Print and shaded views of the part. All mm, measured from the part's lowest x, y and z. A direction names the side the tool comes from. Round coordinates to 2 decimals unless told otherwise and drop trailing zeros. Write each loop counter-clockwise with the first axis right and the second up, starting at its lowest first coordinate (ties: lowest second). Pieces come first, ordered by that corner, then holes. Notation, with made-up numbers: M -4,7.5 L 11,7.5 A20 cw 11,41.5 Z; hole C 30.5,26 d8. An arc over 180 degrees is marked long. Write item = value, one per line. Start each with the question number.
Q1. Tool access for the marked faces 1 and 2: list every direction of +Z, -Z, +X, -X, +Y, -Y with a clear straight run to the whole face (end or side of a thin tool).
Q2. Drop flat-ended pins along their axis: P1, Ø2, axis at x = 270, y = 35.5, coming from the -Z side; P2, Ø12, axis at x = 170, y = 78.5, coming from the -Z side; P3, Ø13.5, axis at x = 363.5, y = 60.5, coming from the +Z side; P4, Ø10, axis at x = 107, z = 97.5, coming from the +Y side. Give the stop position or say it passes through.
Q3. Band-saw the part on D-D on z = 34.5. Write the cut outline in (x, y), plus the area to 3 significant figures.
Q4. Band-saw the part on C-C on x = 385. Write the cut outline in (y, z), plus the area to 3 significant figures.
Q5. Band-saw the part on A-A on z = 60. Write the cut outline in (x, y), plus the area to 3 significant figures.
Q6. Probe L1, parallel to X at y = 36, z = 5.5; L2, parallel to X at y = 49, z = 74; L3, parallel to Y at x = 50.5, z = 58. List the from-to ranges inside material, lowest first.
Q7. Band-saw the part on B-B on y = 60. Write the cut outline in (x, z).
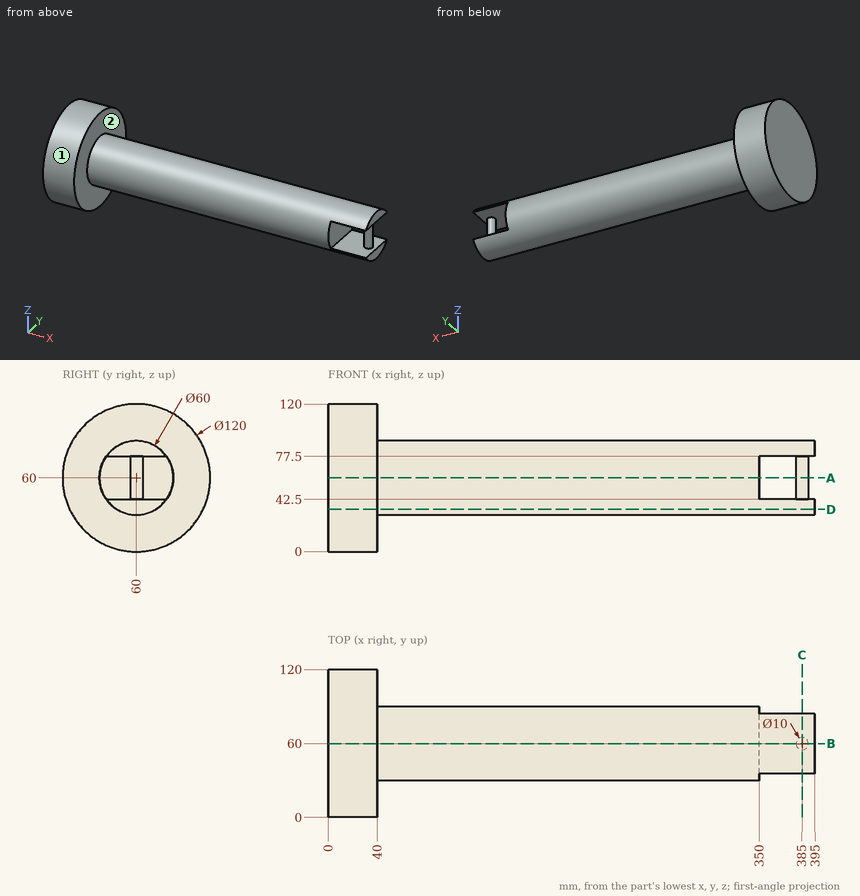
Conclusion:
q1.face_1 = +X, -X
q1.face_2 = +X
q2.P1 = 41.35
q2.P2 = 32.73
q2.P3 = 90
q2.P4 = through
q3.outline = M 0,5.69 L 40,5.69 L 40,44.2 L 395,44.2 L 395,75.8 L 40,75.8 L 40,114.31 L 0,114.31 Z
q3.area = 15,600 mm^2
q4.outline = M 35.63,42.5 A30 ccw 84.37,42.5 L 65,42.5 L 65,77.5 L 84.37,77.5 A30 ccw 35.63,77.5 L 55,77.5 L 55,42.5 Z
q4.area = 1,200 mm^2
q5.outline = M 0,0 L 40,0 L 40,30 L 350,30 L 350,90 L 40,90 L 40,120 L 0,120 Z; C 385,60 d10
q5.area = 23,500 mm^2
q6.L1 = 0 to 40
q6.L2 = 0 to 350
q6.L3 = 30.07 to 89.93
q7.outline = M 0,0 L 40,0 L 40,30 L 395,30 L 395,42.5 L 390,42.5 L 390,77.5 L 395,77.5 L 395,90 L 40,90 L 40,120 L 0,120 Z; hole M 350,42.5 L 380,42.5 L 380,77.5 L 350,77.5 Z
